Check sheet for the drawn part. Datum: minimum x, y, z corner. Units: mm. A direction names the side the tool comes from. Coordinates: 2 decimals unless noted, no trailing zeros. Write each loop counter-clockwise with the first axis right and the second up, starting at its lowest first coordinate (ties: lowest second). Pieces come first, ordered by that corner, then holes. Notation, with made-up numbers: (-13, 47.5) - (23, 47.5) arc R15 ccw to (23, 59.5) - close; hole circle Ø3 at (-34, -23). An arc over 180 degrees is marked (long way). Write each question's results on one line, items separated by ' | '.
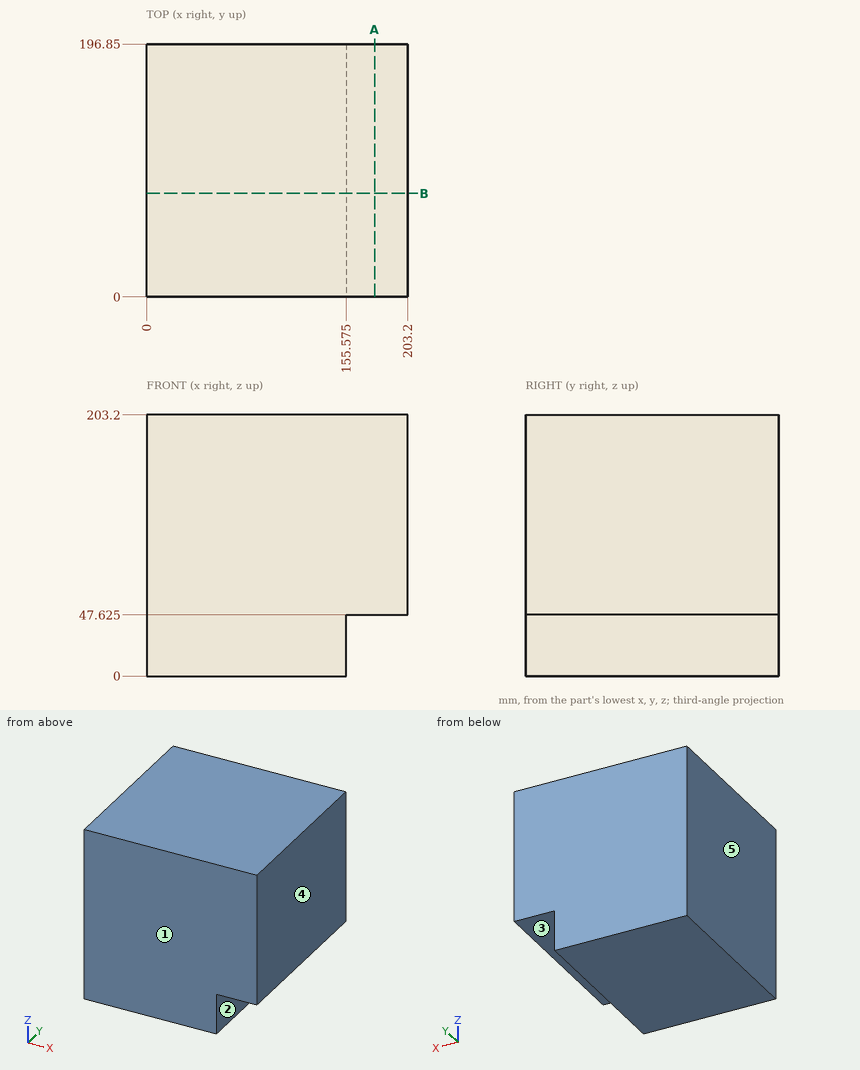
1. Access from +Z, -Z, +X, -X, +Y, -Y to the whole of each face (thin tool, end or side, straight path). Record for the marked faces 1 and 2.
Values follow:
face 1: +Z, -Z, +X, -X, -Y | face 2: -Z, +X, +Y, -Y
2. Draft check along X on the marked faces 3, 4 and 5. Enter one of: pulls with the +X half, pulls with the -X half, needs draft (parallel to the pull), parting line crosses it, or undercut.
Values follow:
face 3: needs draft | face 4: pulls with the +X half | face 5: pulls with the -X half
3. Sectioned sample at A-A (x = 177.5). Record the cut outline in (y, z) (3 decimals).
Values follow:
outline: (0, 47.625) - (196.85, 47.625) - (196.85, 203.2) - (0, 203.2) - close
4. Material ranges on L1, parallel to Z at x = 194, y = 63.5 (3 decimals); L2, parallel to X at y = 129, z = 9 (3 decimals), recorded low to high. Write a range as [from, to].
Values follow:
L1: z = [47.625, 203.2] | L2: x = [0, 155.575]
5. Sectioned sample at B-B (y = 80.5). Record the cut outline in (x, z) (3 decimals), then the cut area to 3 significant figures.
Values follow:
outline: (0, 0) - (155.575, 0) - (155.575, 47.625) - (203.2, 47.625) - (203.2, 203.2) - (0, 203.2) - close | area: 39,000 mm^2
